Autodesk Inventor part; units mm, degrees
ref_plane "YZ Plane" through (0, 0, 0) normal (1, 0, 0) x (0, 1, 0)
ref_plane "XZ Plane" through (0, 0, 0) normal (0, 1, 0) x (-1, 0, 0)
ref_plane "XY Plane" through (0, 0, 0) normal (0, 0, 1) x (1, 0, 0)
sketch "Sketch1" plane through (0, 0, 0) normal (0, 1, 0) x (-1, 0, 0)
  line L0 (-40, 50) -> (40, 50)
  line L1 (40, 50) -> (40, -50)
  line L2 (40, -50) -> (-40, -50)
  line L3 (-40, -50) -> (-40, 50)
  line L4 (-40, 50) -> (40, -50) construction
  line L5 (40, 50) -> (-40, -50) construction
  point P0 (0, 0)
  dimension "d0" = 100
  dimension "d1" = 80
extrude "Extrusion1" add sketch "Sketch1" along normal blind 10
sketch "Sketch2" plane through (0, 10, 0) normal (0, 1, 0) x (1, 0, 0)
  line L0 (-40, -50) -> (40, -50)
  line L1 (40, -50) -> (25, -50)
  line L2 (25, -50) -> (25, -35)
  line L3 (25, -35) -> (40, -35)
  line L4 (40, -35) -> (40, -50)
  line L5 (25, -35) -> (35, -35)
  line L6 (35, -35) -> (35, -45)
  line L7 (35, -45) -> (25, -45)
  line L8 (25, -45) -> (25, -35)
  point P0 (0, 0)
  dimension "d4" = 15
  dimension "d5" = 15
  dimension "d6" = 10
  dimension "d7" = 10
extrude "Extrusion2" add sketch "Sketch2" along normal blind 120 contours L2 L7 L6 L3 L4 L0
mirror "Mirror1" about plane through (0, 0, 0) normal (0, 0, 1) of "Extrusion2"
mirror "Mirror2" about plane through (0, 0, 0) normal (1, 0, 0) of "Extrusion2", "Mirror1"
sketch "Sketch3" plane through (0, 10, 0) normal (0, 1, 0) x (1, 0, 0)
  line L0 (-25.02, -38.04) -> (23.02, -38.04)
  line L1 (23.02, -38.04) -> (23.02, 12)
  line L2 (23.02, 12) -> (-25.02, 12)
  line L3 (-25.02, 12) -> (-25.02, -38.04)
  line L4 (25, 50) -> (-25, 50)
  point P0 (0, 0)
  dimension "d10" = 48.04
  dimension "d11" = 50.04
  dimension "d13" = 25.02
  dimension "d14" = 38
extrude "Extrusion3" cut sketch "Sketch3" against normal blind 5.04
sketch "Sketch4" plane through (0, 10, 0) normal (0, 1, 0) x (1, 0, 0)
  circle A0 centre (0, 30) radius 7.52
  line L0 (25, 50) -> (-25, 50)
  line L1 (-40, 35) -> (-40, -35)
  point P0 (0, 0)
  dimension "d17" = 15.04
  dimension "d18" = 20
  dimension "d19" = 40
extrude "Extrusion4" cut sketch "Sketch4" against normal blind 5.04
sketch "Sketch6" plane through (-40, 0, 50) normal (0, 0, 1) x (1, 0, 0)
  line L0 (63.02, 10) -> (14.98, 10)
  line L1 (65, 10) -> (65, 130)
  line L2 (35, 5) -> (45, 5)
  line L3 (45, 5) -> (45, 15)
  line L4 (45, 15) -> (35, 15)
  line L5 (35, 15) -> (35, 5)
  line L6 (35, 5) -> (45, 15) construction
  line L7 (45, 5) -> (35, 15) construction
  point P0 (40, 0)
  dimension "d24" = 10
  dimension "d25" = 10
  dimension "d26" = 20
  dimension "d27" = 5
extrude "Extrusion5" cut sketch "Sketch6" against normal blind 15
Read the model definition and answer for the solid it produces. Units are mm, in the model's axes. A direction names the side the tool comes from. Give positions to 0.01 mm unless a question says otherwise; leave off trailing zeros. Write each loop counter-clockwise with the first axis right and the second up, starting at its lowest first coordinate (ties: lowest second). Pieces come first, ordered by that corner, then holes. Notation, with made-up numbers: (25.5, 39) - (72.5, 39) arc R16 ccw to (72.5, 55) - close; hole circle Ø1 at (20.25, 40.5). An arc over 180 degrees is marked (long way). Answer in a Markdown table with one row per item. Add a question column.
Item 1: Find the intervals of material crossed by L1, parallel to Z at x = -33.5, y = 85.5; L2, parallel to X at y = 8.4, z = -30; L3, parallel to Z at x = 0, y = 8, in increasing order.
Item 2: Section B-B, the plane z = -30 is taken. Write down the section's boundary in (x, y).
Item 3: Flat-ended cylindrical pins translate along their axes: P1, Ø1, axis at x = 19.5, z = -25.5, coming from the +Y side; P2, Ø3, axis at x = 4, z = 16.5, coming from the +Y side. Find the tip coordinate at first contact, or state that the pin passes through.
Item 4: Determine the mould class of faces 1 (the face through (-40, 55, 37)), 2 (the face through (-35, 69, -40)) for opening direction Z: pulls with the +Z half, pulls with the -Z half, needs draft (parallel to the pull), parting line crosses it, or undercut.
Item 5: Section A-A, the plane y = 82 is taken. Write down the section's boundary in (x, z).
Item 6: A tool of negligible diameter and unlimited length cuts with its end or side. For faces 3 (the face through (-30, 69, -45)), 4 (the face through (25, 69, 48)), 5 (the face through (36, 130, 44)), 6 (the face through (-38, 69, 35)), from which of +Z, -Z, +X, -X, +Y, -Y can it reach the whole face along a straight path? Write none if from no direction.
Item 7: Section C-C, the plane x = 0 is taken. Write down the section's boundary in (y, z).
Item 8: Section D-D, the plane x = 20 is taken. Write down the section's boundary in (y, z), and give its area (3 significant figures).
Recorded:
| question | item | result |
|---|---|---|
| 1 | L1 | z = -50 to -45, 45 to 50 |
| 1 | L2 | x = -40 to -7.52, 7.52 to 40 |
| 1 | L3 | z = -50 to -37.52, -22.48 to -12 |
| 2 | outline | (-40, 0) - (40, 0) - (40, 10) - (7.52, 10) - (7.52, 4.96) - (-7.52, 4.96) - (-7.52, 10) - (-40, 10) - close |
| 3 | P1 | stops at y = 10 |
| 3 | P2 | stops at y = 4.96 |
| 4 | face 1 | needs draft |
| 4 | face 2 | undercut |
| 5 | outline | (-40, -50) - (-25, -50) - (-25, -45) - (-35, -45) - (-35, -35) - (-40, -35) - close; (-40, 35) - (-35, 35) - (-35, 45) - (-25, 45) - (-25, 50) - (-40, 50) - close; (25, -50) - (40, -50) - (40, -35) - (35, -35) - (35, -45) - (25, -45) - close; (25, 45) - (35, 45) - (35, 35) - (40, 35) - (40, 50) - (25, 50) - close |
| 6 | face 3 | +Y |
| 6 | face 4 | +Z, -Z, +Y |
| 6 | face 5 | +Z, -Z, +X, -X, +Y |
| 6 | face 6 | +X, -X, +Y |
| 7 | outline | (0, -50) - (10, -50) - (10, -37.52) - (4.96, -37.52) - (4.96, -22.48) - (10, -22.48) - (10, -12) - (4.96, -12) - (4.96, 38.04) - (5, 38.04) - (5, 50) - (0, 50) - close |
| 8 | outline | (0, -50) - (10, -50) - (10, -12) - (4.96, -12) - (4.96, 38.04) - (10, 38.04) - (10, 50) - (0, 50) - close |
| 8 | area | 748 mm2 |
